Answer from the drawing. Dimensions are ordinates in mm from the lowest x, y and z of the part. Coordinates: 2 decimals unless noted, no trailing zeros. Order: outer loops, then holes, each group sorted by start corner. A loop starts at its lowest first (then second) coordinate and runs counter-clockwise, first axis right, second up. Notation, with made-up numbers: (44.5, -19.5) - (77.5, -19.5) arc R37 cw to (77.5, 19.5) - close; hole circle Ø10 at (46.5, 41). An arc over 180 degrees is marked (long way). Answer as a JSON object with one key per item and string values. Group by question number.
1) Find the intervals of material crossed by line 1 along X through (y, z) = (19, 22) (1 decimal); line 2 along Y through (x, z) = (19.05, 15.5) (1 decimal); line 3 along Y through (x, z) = (18, 29), in increasing order.
2) Section D-D (x = 31.5) is taken. Give the vertices of the cut face in (y, z).
3) Section A-A (x = 19.05) is taken. Give the vertices of the cut face in (y, z) (1 decimal), plus the area to 3 significant figures.
4) Each of these flat-tipped pins is pushed along its axis until it touches: P1, Ø12, axis at x = 13.5, z = 10, coming from the +Y side; P2, Ø3, axis at y = 22, z = 5, coming from the -X side; P3, Ø10, axis at x = 6, z = 18.5, coming from the -Y side. Where does it stop, or does it pass through?
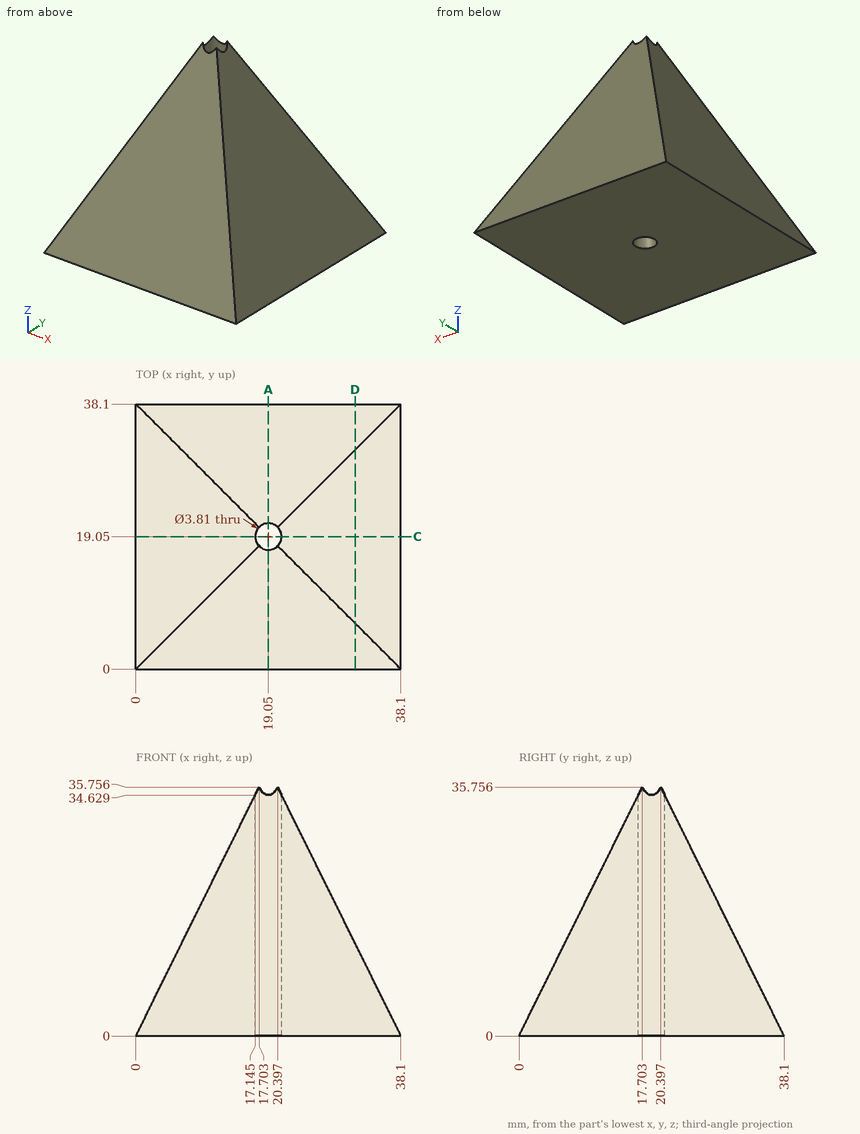
Report:
{
 "1": {"line 1": "x = 10.9 to 17.1, 21 to 27.2", "line 2": "y = 7.7 to 17.1, 21 to 30.4", "line 3": "y = 14.36 to 17.46, 20.64 to 23.74"},
 "2": {"outline": "(0, 0) - (38.1, 0) - (31.5, 13.33) - (6.6, 13.33) - close"},
 "3": {"outline": "(0, 0) - (17.1, 0) - (17.1, 34.6) - close; (21, 0) - (38.1, 0) - (21, 34.6) - close", "area": "594 mm²"},
 "4": {"P1": "stops at y = 36.12", "P2": "stops at x = 1.73", "P3": "stops at y = 6.71"}
}
